Autodesk Inventor part; units mm, degrees
ref_plane "Diagonal Plane" through (-4.7625, 1.5875, 0) normal (-0.7071068, 0.7071068, 0) x (0, 0, 1)
ref_plane "YZ Plane" through (0, 0, 0) normal (1, 0, 0) x (0, 1, 0)
ref_plane "XZ Plane" through (0, 0, 0) normal (0, 1, 0) x (-1, 0, 0)
sketch "Sketch1" plane through (0, 0, 0) normal (0, 1, 0) x (-1, 0, 0)
  line L0 (-6.35, 0) -> (6.35, 0)
  line L1 (6.35, 0) -> (6.35, -12.7)
  line L2 (6.35, -12.7) -> (-6.35, -12.7)
  line L3 (-6.35, -12.7) -> (-6.35, 0)
  line L4 (6.35, 0) -> (-6.35, -12.7) construction
  point P0 (0, 0)
  point P1 (0, 0)
  dimension "d0" = 12.7
  dimension "d1" = 12.7
extrude "Plate1" add sketch "Sketch1" along normal blind 1.5875
sketch "Sketch2" plane through (-4.7625, 0, 0) normal (-1, 0, 0) x (0, -1, 0)
  line L0 (0, -12.7) -> (0, 0)
  line L1 (0, 0) -> (-12.7, 0)
  line L2 (-12.7, 0) -> (-12.7, -12.7)
  line L3 (-12.7, -12.7) -> (0, -12.7)
edge flange "Flanges" height 12.7 angle 90 thickness 1.5875 bend radius 0.7937 thickness toward (-1, 0, 0) relief tear relief width 1.5875 relief depth 0.7937 edges at (-6.35, 1.5875, -6.35) wall of the first edge with corners at (-4.7625, 0, -12.7) (-4.7625, 0, 0) (-4.7625, 12.7, 0) (-4.7625, 12.7, -12.7)
bend "Bend1"
corner "Corner1"
sketch "Sketch8" plane through (0, 0, 0) normal (0, -1, 0) x (1, 0, 0)
  line L0 (6.35, 0) -> (-3.9687, 0) construction
  line L1 (2.9718, -4.0386) -> (-0.635, -4.0386)
  line L2 (-1.143, -4.5466) -> (-1.143, -8.1534)
  line L3 (-0.635, -8.6614) -> (2.9718, -8.6614)
  line L4 (3.4798, -8.1534) -> (3.4798, -4.5466)
  arc A0 (3.4798, -4.5466) -> (2.9718, -4.0386) centre (2.9718, -4.5466) ccw
  arc A1 (2.9718, -8.6614) -> (3.4798, -8.1534) centre (2.9718, -8.1534) ccw
  arc A2 (-1.143, -8.1534) -> (-0.635, -8.6614) centre (-0.635, -8.1534) ccw
  arc A3 (-0.635, -4.0386) -> (-1.143, -4.5466) centre (-0.635, -4.5466) ccw
  line L5 (2.9718, -4.5466) -> (-0.635, -8.1534) construction
  line L6 (6.35, -12.7) -> (6.35, 0) construction
  point P0 (0, 0)
  point P1 (-1.143, -8.6614)
  point P2 (3.4798, -8.6614)
  point P3 (12.7, 0)
  point P4 (1.1684, -6.35)
  dimension "d49" = 4.6228
  dimension "d50" = 0.508
  dimension "d52" = 6.35
  dimension "d123" = 5.1816
extrude "Body Stamp" cut sketch "Sketch8" against normal blind 1.5875
sketch "Sketch9" plane through (0, 0, 0) normal (0, -1, 0) x (1, 0, 0)
  arc A0 (3.4798, -4.5466) -> (2.9718, -4.0386) centre (2.9718, -4.5466) ccw construction
  arc A1 (-1.143, -8.1534) -> (-0.635, -8.6614) centre (-0.635, -8.1534) ccw construction
  line L0 (2.9718, -4.5466) -> (-0.635, -8.1534) construction
  circle A2 centre (1.1684, -6.35) radius 2.1844
  point P0 (0, 0)
  dimension "d55" = 4.3688
surface extrude "Body Circle" sketch "Sketch9" against normal up to surface (1.5875 mm away) shown yes curves A2
pattern_sketch "Body Pattern" of "Body Stamp", "Body Circle" from (1.1684, 0, -6.35) copies at (1.1684, 0, -19.05) at (1.1684, 0, -31.75) at (1.1684, 0, -44.45) at (1.1684, 0, -57.15) at (1.1684, 0, -69.85) at (1.1684, 0, -82.55) at (1.1684, 0, -95.25) at (1.1684, 0, -107.95) at (1.1684, 0, -120.65) at (1.1684, 0, -133.35) at (1.1684, 0, -146.05) at (1.1684, 0, -158.75) at (1.1684, 0, -171.45) at (1.1684, 0, -184.15) at (1.1684, 0, -196.85) at (1.1684, 0, -209.55) at (1.1684, 0, -222.25) at (1.1684, 0, -234.95) at (1.1684, 0, -247.65) at (1.1684, 0, -260.35) at (1.1684, 0, -273.05) at (1.1684, 0, -285.75) at (1.1684, 0, -298.45) at (1.1684, 0, -311.15) at (1.1684, 0, -323.85) at (1.1684, 0, -336.55) at (1.1684, 0, -349.25) at (1.1684, 0, -361.95) at (1.1684, 0, -374.65) at (1.1684, 0, -387.35) at (1.1684, 0, -400.05) at (1.1684, 0, -412.75) at (1.1684, 0, -425.45) at (1.1684, 0, -438.15)
sketch "Arc Length" plane through (19.05, 2.3812, 0) normal (0, 0, 1) x (1, 0, 0)
  line L0 (-25.4, 0) -> (-23.8125, 0)
  arc A0 (-25.4, 0) -> (-23.0187, -2.3813) centre (-23.0187, 0) ccw
  line L1 (-23.0187, -0.7938) -> (-23.0187, -2.3813)
  arc A1 (-23.8125, 0) -> (-23.0187, -0.7938) centre (-23.0187, 0) ccw
  point P0 (-19.05, -2.3812)
  dimension "d126" = 1.2468
  dimension "d127" = 3.7405
sketch "Sketch13" plane through (-6.35, 0, 431.8) normal (1, 0, 0) x (0, 0, -1)
  line L0 (493.268, 12.7) -> (495.3, 10.668)
  line L1 (495.3, 10.668) -> (497.332, 12.7)
  line L2 (493.268, 12.7) -> (497.332, 12.7)
  line L3 (495.3, 3.3973) -> (493.0372, 1.1344)
  line L4 (493.0372, 1.1344) -> (495.3, -1.1284)
  line L5 (495.3, -1.1284) -> (497.5628, 1.1344)
  line L6 (497.5628, 1.1344) -> (495.3, 3.3973)
  line L7 (495.3, 3.3973) -> (495.3, -1.1284) construction
  line L8 (495.3, 10.668) -> (495.3, 3.3973) construction
  line L9 (444.5, 12.7) -> (431.8, 12.7)
  line L10 (444.5, 2.3813) -> (431.8, 2.3813) construction
  line L11 (431.8, 12.7) -> (431.8, 2.3813) construction
  point P0 (444.5, -11.9062)
  point P1 (431.8, 0)
  dimension "d86" = 4.5256
  dimension "d128" = 2.032
  dimension "d129" = 1.016
  dimension "d130" = 63.5
feature "Notch" [suppressed]
pattern_linear "Notch Pattern" [suppressed]
ref_plane "Diagonal Plane" through (-4.7625, 1.5875, 0) normal (-0.7071068, 0.7071068, 0) x (0, 0, 1)
mirror "Everything Mirrored" about plane through (-4.7625, 1.5875, 0) normal (-0.7071068, 0.7071068, 0) of "Body Stamp", "Body Circle", "Body Pattern"
chamfer "End Chamfer" distance 1.016 angle 45 4 edges at (-5.5562, 12.7, -12.7) (-5.5562, 12.7, 0) (6.35, 0.7937, 0) (6.35, 0.7937, -12.7)
sketch "Sketch17" plane through (-6.35, 2.3813, -12.7) normal (-1, 0, 0) x (0, 0, 1)
  line L0 (12.7, 9.3028) -> (12.7, 0) construction
  line L1 (0, 0) -> (0, 9.3027) construction
  line L2 (1.016, 10.3187) -> (11.684, 10.3188) construction
  line L3 (0, 2.7171) -> (4.577, 8.1963)
  line L4 (6.35, 1.587) -> (6.35, 9.3027) construction
  line L5 (12.7, 2.7171) -> (8.123, 8.1963)
  line L6 (4.577, 8.1963) -> (8.123, 8.1963)
  line L7 (0, 2.7171) -> (0, 10.3187)
  line L8 (0, 10.3187) -> (12.7, 10.3187)
  line L9 (12.7, 10.3187) -> (12.7, 2.7171)
  point P0 (12.7, -2.3812)
extrude "Extrusion2" cut sketch "Sketch17" against normal blind 1.5875
sketch "Body Pattern Sketch" plane through (0, 0, 0) normal (0, -1, 0) x (1, 0, 0)
  line L0 (1.1684, -6.35) -> (1.1684, 0) construction
  circle A0 centre (1.1684, -6.35) radius 2.1844 construction
  point P0 (1.1684, -19.05)
  point P1 (1.1684, -31.75)
  point P2 (1.1684, -44.45)
  point P3 (1.1684, -57.15)
  point P4 (1.1684, -69.85)
  point P5 (1.1684, -82.55)
  point P6 (1.1684, -95.25)
  point P7 (1.1684, -107.95)
  point P8 (1.1684, -120.65)
  point P9 (1.1684, -133.35)
  point P10 (1.1684, -146.05)
  point P11 (1.1684, -158.75)
  point P12 (1.1684, -171.45)
  point P13 (1.1684, -184.15)
  point P14 (1.1684, -196.85)
  point P15 (1.1684, -209.55)
  point P16 (1.1684, -222.25)
  point P17 (1.1684, -234.95)
  point P18 (1.1684, -247.65)
  point P19 (1.1684, -260.35)
  point P20 (1.1684, -273.05)
  point P21 (1.1684, -285.75)
  point P22 (1.1684, -298.45)
  point P23 (1.1684, -311.15)
  point P24 (1.1684, -323.85)
  point P25 (1.1684, -336.55)
  point P26 (1.1684, -349.25)
  point P27 (1.1684, -361.95)
  point P28 (1.1684, -374.65)
  point P29 (1.1684, -387.35)
  point P30 (1.1684, -400.05)
  point P31 (1.1684, -412.75)
  point P32 (1.1684, -425.45)
  point P33 (1.1684, -438.15)
  dimension "d133" = 12.7
equation "\"d1\" = 1.27 * Length"
equation "\"d53\" = Thickness"
equation "\"d89\" = Thickness"
equation "\"d2\" = Thickness"
equation "\"d3\" = BendReliefWidth"
equation "\"d4\" = BendReliefDepth"
equation "\"d5\" = MinimumRemnant"
equation "\"d6\" = TransitionRadius"
equation "\"d10\" = CornerReliefSize"
equation "\"d11\" = GapSize"
equation "\"d12\" = JacobiRadiusSize"
equation "\"BendRadius\" = Thickness"
equation "\"BendReliefWidth\" = Thickness"
equation "\"BendReliefDepth\" = 0.5 * Thickness"
equation "\"CornerReliefSize\" = 4 * Thickness"
equation "\"MinimumRemnant\" = 2 * Thickness"
equation "\"TransitionRadius\" = BendRadius"
equation "\"JacobiRadiusSize\" = BendRadius"
equation "\"GapSize\" = Thickness"
properties part number "Alu C 1x2x1x35"
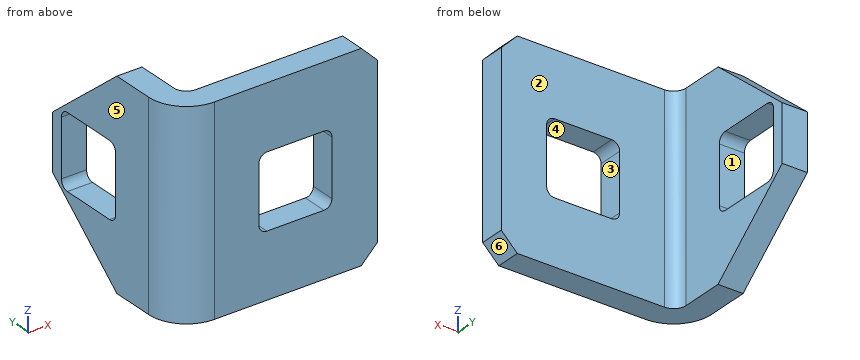
Verification items for the finished model (mm, model axes). Face numbers are marked on the shaded views. A direction names the side the tool comes from. Coordinates: 2 decimals unless noted, no trailing zeros. Order: outer loops, then holes, each group sorted by start corner. A loop starts at its lowest first (then second) coordinate and runs counter-clockwise, first axis right, second up. Notation, with made-up numbers: (46.5, -36.5) -> (89.5, -36.5) arc R15 ccw to (89.5, -26.5) -> close; hole circle Ø1 at (9, -22.5). An arc over 180 degrees is marked (long way). Put each result on its own line as item: value. Start each with the question number.
1. Cross-section at A-A, the plane x = 0. Record the boundary of the cut face in (y, z), then the cut area to 3 significant figures.
2. Cross-section at D-D, the plane z = -3. Record the boundary of the cut face in (x, y).
3. Cross-section at B-B, the plane z = -5.75. Record the boundary of the cut face in (x, y).
4. Cross-section at C-C, the plane y = 8.25. Record the boundary of the cut face in (x, z).
5. Access from +Z, -Z, +X, -X, +Y, -Y to the whole of each face (thin tool, end or side, straight path). Record for the marked faces 1, 2 and 3.
6. Material ranges on L1, parallel to Y at x = 5, z = -12; L2, parallel to X at y = 4.5, z = -11.75; L3, parallel to Y at x = -5.25, z = -7.5, recorded low to high. Write a range as [from, to].
7. Go/stop test with flat-tipped pins: pin 1 Ø4 at (y, z) = (7.5, -5) entering from +X; pin 2 Ø1.3 at (x, z) = (-5.5, -5.5) entering from -Y; pin 3 Ø2 at (x, z) = (-3, -4.5) entering from +Y. Record where each tip stops, or that it passes through.
8. Mould release check, pull along Z, two halves, no side actions. Record for the marked faces 4, 5 and 6: released by +Z, released by -Z, zero draft, split by the parting line, or undercut.
Computed:
1. outline: (0, -12.7) -> (1.59, -12.7) -> (1.59, -8.66) -> (0, -8.66) -> close; (0, -4.04) -> (1.59, -4.04) -> (1.59, 0) -> (0, 0) -> close
1. area: 12.8 mm2
2. outline: (-6.35, 2.38) arc R2.38 ccw to (-3.97, 0) -> (6.35, 0) -> (6.35, 1.59) -> (-3.97, 1.59) arc R0.79 cw to (-4.76, 2.38) -> (-4.76, 8.69) -> (-6.35, 8.69) -> close
3. outline: (-6.35, 2.38) arc R2.38 ccw to (-3.97, 0) -> (-1.14, 0) -> (-1.14, 1.59) -> (-3.97, 1.59) arc R0.79 cw to (-4.76, 2.38) -> (-4.76, 5.21) -> (-6.35, 5.21) -> close; (-6.35, 9.83) -> (-4.76, 9.83) -> (-4.76, 10.58) -> (-6.35, 10.58) -> close; (3.48, 0) -> (6.35, 0) -> (6.35, 1.59) -> (3.48, 1.59) -> close
4. outline: (-6.35, -10.07) -> (-4.76, -10.07) -> (-4.76, -8.66) -> (-6.35, -8.66) -> close; (-6.35, -4.04) -> (-4.76, -4.04) -> (-4.76, -2.63) -> (-6.35, -2.63) -> close
5. face 1: +X, -X
5. face 2: +Z, -Z, +X, +Y
5. face 3: +Y, -Y
6. L1: [0, 1.59]
6. L2: [-6.35, -4.76]
6. L3: [0.37, 5.21], [9.83, 10.58]
7. pin 1: x = -4.76
7. pin 2: y = 0.17
7. pin 3: y = 1.59
8. face 4: undercut
8. face 5: zero draft
8. face 6: released by -Z
